The listing builds one solid part. Answer for the finished solid, in the listing's coordinates (mm). A direction names the side the tool comes from. Round coordinates to 2 decimals unless told otherwise and drop trailing zeros. Write each loop counter-clockwise with the first axis right and the second up, starting at its lowest first coordinate (ties: lowest second). Pieces come first, ordered by that corner, then holes.
from build123d import *

# Parameters (mm, degrees)
SKETCH1_R           = 189.992
BOSS_EXTRUDE1_DEPTH = 210.058
FILLET1_R           = 12.7
SHELL1_T            = -2.5
SKETCH2_W           = 88.646
SKETCH2_H           = 12.7
BOSS_EXTRUDE2_DEPTH = 32.258
CIRPATTERN1_COUNT   = 20


with BuildPart() as part:
    # Sketch1 → Boss-Extrude1 (new body)
    with BuildSketch(Plane(origin=(0, 0, 0), x_dir=(1, 0, 0), z_dir=(0, 1, 0))):
        with Locations(Location((0, 0, 0), (0, 0, 90))):
            Circle(SKETCH1_R)
    extrude(amount=BOSS_EXTRUDE1_DEPTH)

    # Fillet1
    fillet1_edges = [part.edges().sort_by_distance(p)[0] for p in [
        (0, 0, 189.992),
    ]]
    fillet(fillet1_edges, radius=FILLET1_R)

    # Shell1
    shell1_openings = [part.faces().sort_by_distance(p)[0] for p in [
        (0, 210.058, 0),
    ]]
    offset(amount=SHELL1_T, openings=shell1_openings, kind=Kind.INTERSECTION)

    # Sketch2 → Boss-Extrude2 (add)
    with BuildSketch(Plane(origin=(0, 0, 0), x_dir=(-1, 0, 0), z_dir=(0, -1, 0))):
        with Locations((132.969, 1.507022024)):
            Rectangle(SKETCH2_W, SKETCH2_H)
    boss_extrude2 = extrude(amount=BOSS_EXTRUDE2_DEPTH)

    # CirPattern1: Boss-Extrude2 ×20 about axis
    cirpattern1_axis = Axis((0, 0, 0), (0, 1, 0))
    for i in range(1, CIRPATTERN1_COUNT):
        add(boss_extrude2.rotate(cirpattern1_axis, i * 360 / CIRPATTERN1_COUNT))


solid = part.part
1. A tool of negligible diameter and unlimited length cuts with its end or side. For faces 4 (the face through (169.053, -15.903, -53.438)), 5 (the face through (73.874, -15.903, -109.919)), 6 (the face through (-7.857, -16, 132)), from which of +Z, -Z, +X, -X, +Y, -Y can it reach the whole face along a straight path? Write none if from no direction.
Geometry says:
face 4: -Z, +X, -Y
face 5: -Y
face 6: +Z, -Z, -Y
2. Given pin 1 (2.5 mm diameter, centred on x = 142.5, z = -106, fed in from +Y); pin 2 (2.5 mm diameter, centred on x = 146, z = -99.5, fed in from +Y); pin 3 (10 mm diameter, centred on x = 101.5, y = 34, fed in from -Z), each flat-ended and moving along its own axis, determine where each tip first touches the part or whether it passes through.
Geometry says:
pin 1: stops at y = 2.62
pin 2: stops at y = 2.52
pin 3: stops at z = -163.66
3. Straight lines are drawn through the part: line 1 along Z through (x, y) = (-4, 126); line 2 along Z through (x, y) = (-113.5, -17); line 3 along X through (y, z) = (118, 0). For each, find the intervals that lie inside material, in ascending order.
Geometry says:
line 1: z = -189.95 to -187.45, 187.45 to 189.95
line 2: z = -92.17 to -76.48, -45.14 to -31.79, -7.86 to 4.84, 28.62 to 41.97, 72.75 to 88.45
line 3: x = -189.99 to -187.49, 187.49 to 189.99
4. Section A-A on y = 80.5 is taken. Determine the outline of the cut face in (x, z), plus the area to 3 significant figures.
Geometry says:
outline: circle Ø379.98 at (0, 0); hole circle Ø374.98 at (0, 0)
area: 2,960 mm2
5. For a pull along Z with two mould halves and no side action, classify faces 1 (the face through (109.919, -15.903, 73.874)), 2 (the face through (106, -32.258, 79)), 3 (the face through (56.13, -15.9, -168.18)) as released by +Z, released by -Z, zero draft, split by the parting line, or undercut.
Geometry says:
face 1: undercut
face 2: zero draft
face 3: released by -Z
6. Section B-B on y = -12 is taken. Give the number of separate pieces and of enclosed holes in the cut face, plus the area to 3 significant figures.
Geometry says:
separate pieces: 20
enclosed holes: 0
area: 22,500 mm2
